The listing builds one solid part. Answer for the finished solid, in the listing's coordinates (mm). Coordinates: 2 decimals unless noted, no trailing zeros. Loops run counter-clockwise (first coordinate to the right, second up) from the corner with the lowest first, then second, coordinate; pieces in that order, holes last. Notation, with made-up numbers: M 55.5,35 L 66.5,35 A18 cw 66.5,61 Z; hole C 75,-17 d10. An arc over 180 degrees is marked long. Return JSON: item names as keys, results as strings. Group by question number.
1. Section A-A (y = 0) is taken. Write down the section's boundary in (x, z).
2. Section C-C (z = -15.5) is taken. Write down the section's boundary in (x, y).
3. Given P1, Ø1, axis at y = -3.5, z = -178.5, coming from the +X side; P2, Ø12, axis at x = 1.5, z = -117.5, coming from the +Y side; P3, Ø12, axis at x = -1.5, z = -124, coming from the -Y side, each flat-ended and moving along its own axis, determine where each tip first touches the part or whether it passes through.
4. Section B-B (x = 1) is taken. Write down the section's boundary in (y, z), then the cut area to 3 significant figures.
5. Straight lines are drawn through the part: L1, parallel to Y at x = 0, z = 4; L2, parallel to Y at x = -0.5, z = -70; L3, parallel to Z at x = -10.75, y = 1.75. For each, find the intervals that lie inside material, in ascending order. Write a range as from..to.
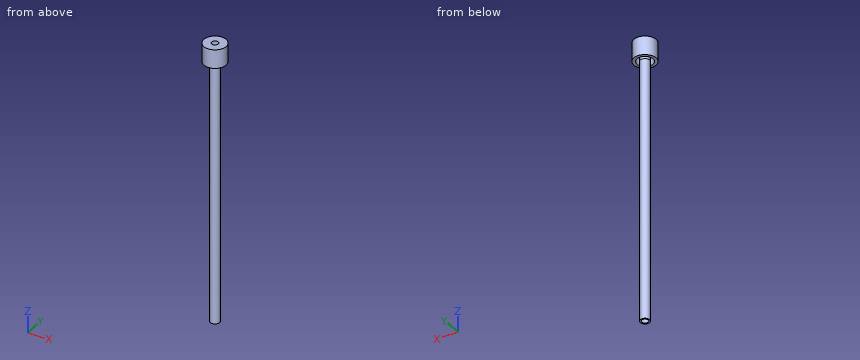
```python
from build123d import *

# Parameters (mm, degrees)
SKETCH1_R           = 12
BOSS_EXTRUDE1_DEPTH = 20
SKETCH2_R           = 8.75
SKETCH2_R_2         = 5
CUT_EXTRUDE1_DEPTH  = 15
SKETCH3_R           = 3.5
CUT_EXTRUDE2_DEPTH  = 27.229754097
SKETCH4_R           = 5
SKETCH4_R_2         = 3.5
BOSS_EXTRUDE2_DEPTH = 280


with BuildPart() as part:
    # Sketch1 → Boss-Extrude1 (new body)
    with BuildSketch(Plane.XY):
        Circle(SKETCH1_R)
    extrude(amount=BOSS_EXTRUDE1_DEPTH)

    # Sketch2 → Cut-Extrude1 (cut)
    with BuildSketch(Plane(origin=(0, 0, 0), x_dir=(-1, 0, 0), z_dir=(0, 0, -1))):
        Circle(SKETCH2_R)
        Circle(SKETCH2_R_2, mode=Mode.SUBTRACT)
    extrude(amount=-CUT_EXTRUDE1_DEPTH, mode=Mode.SUBTRACT)

    # Sketch3 → Cut-Extrude2 (cut, through all)
    with BuildSketch(Plane.XY.offset(20)):
        Circle(SKETCH3_R)
    extrude(amount=-CUT_EXTRUDE2_DEPTH, mode=Mode.SUBTRACT)

    # Sketch4 → Boss-Extrude2 (add)
    with BuildSketch(Plane(origin=(0, 0, 0), x_dir=(-1, 0, 0), z_dir=(0, 0, -1))):
        Circle(SKETCH4_R)
        with Locations(Location((0, 0, 0), (0, 0, 180))):
            Circle(SKETCH4_R_2, mode=Mode.SUBTRACT)
    extrude(amount=BOSS_EXTRUDE2_DEPTH)


solid = part.part
```
Worked out:
{
 "1": {"outline": "M -12,0 L -8.75,0 L -8.75,15 L -5,15 L -5,-280 L -3.5,-280 L -3.5,20 L -12,20 Z; M 3.5,-280 L 5,-280 L 5,15 L 8.75,15 L 8.75,0 L 12,0 L 12,20 L 3.5,20 Z"},
 "2": {"outline": "C 0,0 d10; hole C 0,0 d7"},
 "3": {"P1": "x = 4", "P2": "y = 5", "P3": "y = -5"},
 "4": {"outline": "M -11.96,0 L -8.69,0 L -8.69,15 L -4.9,15 L -4.9,-280 L -3.35,-280 L -3.35,20 L -11.96,20 Z; M 3.35,-280 L 4.9,-280 L 4.9,15 L 8.69,15 L 8.69,0 L 11.96,0 L 11.96,20 L 3.35,20 Z", "area": "1,100 mm^2"},
 "5": {"L1": "-12..-8.75, -5..-3.5, 3.5..5, 8.75..12", "L2": "-4.97..-3.46, 3.46..4.97", "L3": "0..20"}
}
